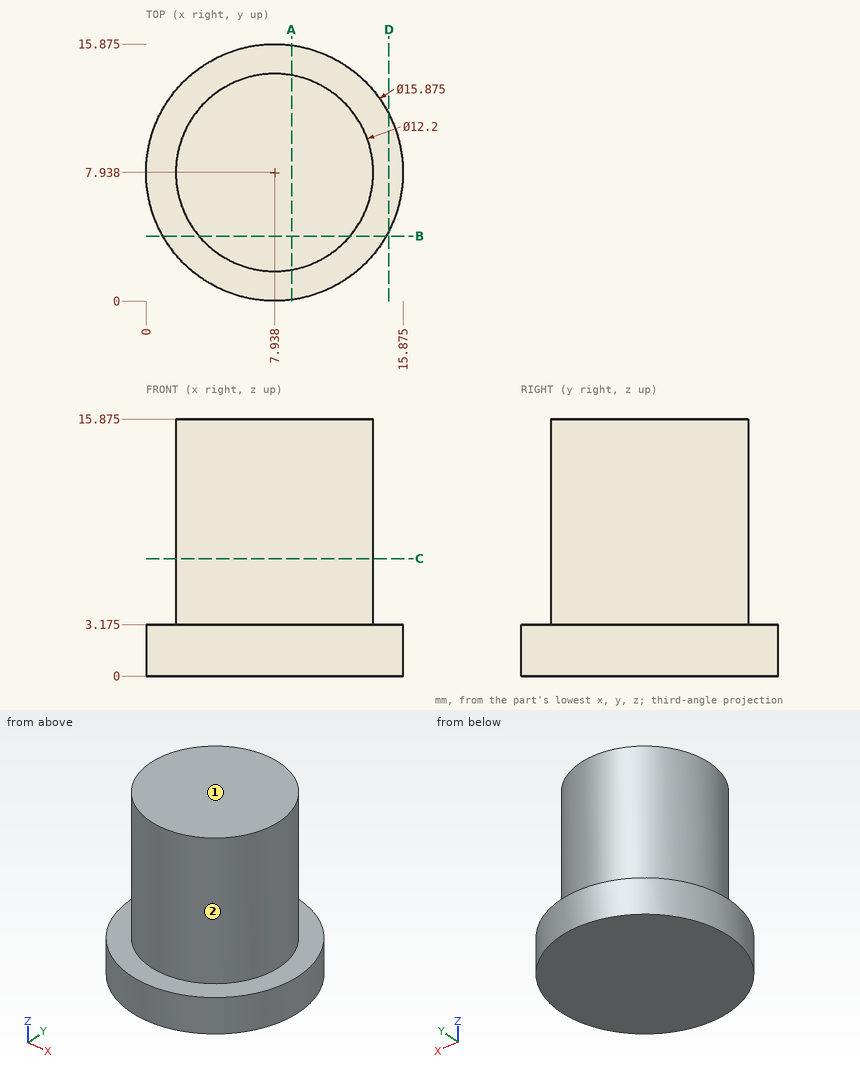
Print and shaded views of the part. All mm, measured from the part's lowest x, y and z. A direction names the side the tool comes from. Give positions to 0.01 mm unless a question says otherwise; leave off trailing zeros. Order: outer loops, then holes, each group sorted by start corner. A loop starts at its lowest first (then second) coordinate and runs counter-clockwise, first axis right, second up. Notation, with made-up numbers: (72.25, 47.25) - (81.25, 47.25) arc R11 ccw to (81.25, 62.25) - close; hole circle Ø6 at (-19.5, -13.75). An arc over 180 degrees is marked (long way). One line per item, written item: value.
Item 1: Wall check: line 1 (Z direction, x = 2.5, y = 5) (1 decimal); line 2 (X direction, y = 7.75, z = 7.5) (1 decimal); line 3 (Y direction, x = 10, z = 4.5) (1 decimal). Give the ranges that are in metal, low to high.
Response values:
line 1: 0 to 3.2
line 2: 1.8 to 14
line 3: 2.2 to 13.7
Item 2: Slice it at D-D (x = 15). List the corners of the cut face in (y, z) (1 decimal).
Response values:
outline: (4.3, 0) - (11.6, 0) - (11.6, 3.2) - (4.3, 3.2) - close
Item 3: Slice it at C-C (z = 7.25). List the corners of the cut face in (x, y), then the cut area to 3 significant figures.
Response values:
outline: circle Ø12.2 at (7.94, 7.94)
area: 117 mm2
Item 4: Slice it at B-B (y = 4). List the corners of the cut face in (x, z) (1 decimal).
Response values:
outline: (1, 0) - (14.8, 0) - (14.8, 3.2) - (12.6, 3.2) - (12.6, 15.9) - (3.3, 15.9) - (3.3, 3.2) - (1, 3.2) - close
Item 5: Tool access for the marked faces 1 and 2: list every direction of +Z, -Z, +X, -X, +Y, -Y with a clear straight run to the whole face (end or side of a thin tool).
Response values:
face 1: +Z, +X, -X, +Y, -Y
face 2: +Z
Item 6: Slice it at A-A (x = 9). List the corners of the cut face in (y, z) (1 decimal).
Response values:
outline: (0.1, 0) - (15.8, 0) - (15.8, 3.2) - (13.9, 3.2) - (13.9, 15.9) - (1.9, 15.9) - (1.9, 3.2) - (0.1, 3.2) - close
Item 7: Pin check, flat tips, straight feed: pin 1 Ø6 at (x, z) = (4, 9.5) entering from -Y; pin 2 Ø1.5 at (y, z) = (11, 7) entering from +X; pin 3 Ø2 at (x, z) = (2.5, 13.5) entering from -Y. Stop position of each tip, or through.
Response values:
pin 1: y = 1.91
pin 2: x = 13.58
pin 3: y = 3.75
